Answer from the drawing. Dimensions are ordinates in mm from the lowest x, y and z of the part. A direction names the side the tool comes from. Give positions to 0.01 mm unless a question says otherwise; leave off trailing zeros. Order: outer loops, then holes, each group sorted by start corner. A loop starts at its lowest first (then second) coordinate and runs counter-clockwise, first axis right, second up. Notation, with made-up numbers: M 73.5,60.5 L 106.5,60.5 A10 ccw 106.5,75.5 Z; hole C -30,52.25 d7. An arc over 180 degrees is marked long. One line per item, written item: value.
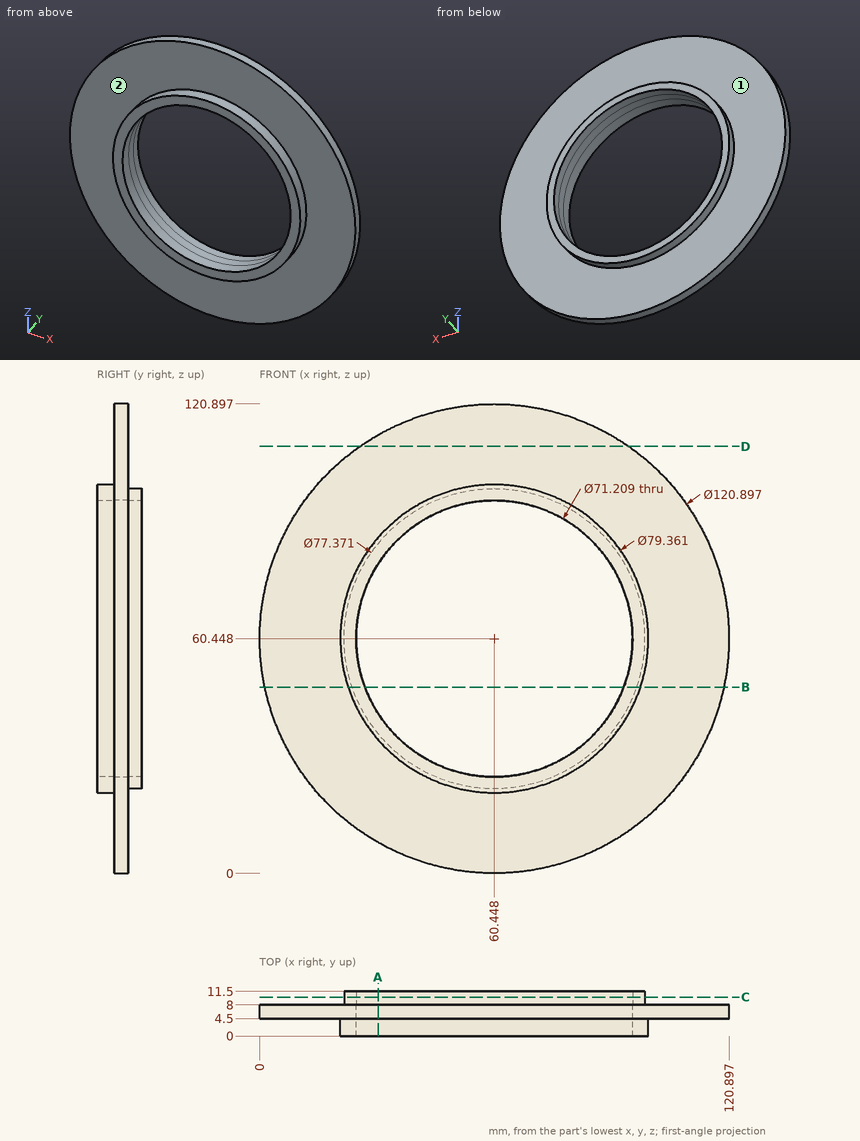
(1) Which of the six approach directions +Z, -Z, +X, -X, +Y, -Y give full straight-line access (tool end or side, diameter ignored) to the marked faces 1 and 2?
Findings:
face 1: +Y
face 2: -Y
(2) Section B-B, the plane z = 48 is taken. Give the vertices of the cut face in (x, y) (1 decimal), then the cut area to 3 significant figures.
Findings:
outline: M 1.3,4.5 L 22.8,4.5 L 22.8,0 L 27.1,0 L 27.1,11.5 L 23.8,11.5 L 23.8,8 L 1.3,8 Z; M 93.8,0 L 98.1,0 L 98.1,4.5 L 119.6,4.5 L 119.6,8 L 97.1,8 L 97.1,11.5 L 93.8,11.5 Z
area: 242 mm^2
(3) Section A-A, the plane x = 30.5 is taken. Give the vertices of the cut face in (y, z) (1 decimal).
Findings:
outline: M 0,34.4 L 4.5,34.4 L 4.5,7.9 L 8,7.9 L 8,36 L 11.5,36 L 11.5,41.2 L 0,41.2 Z; M 0,79.7 L 11.5,79.7 L 11.5,84.9 L 8,84.9 L 8,113 L 4.5,113 L 4.5,86.5 L 0,86.5 Z
(4) Section D-D, the plane z = 110 is taken. Give the vertices of the cut face in (x, y), then the cut area to 3 significant figures.
Findings:
outline: M 25.83,4.5 L 95.07,4.5 L 95.07,8 L 25.83,8 Z
area: 242 mm^2
(5) Section C-C, the plane y = 10 is taken. Give the vertices of the cut face in (x, z) (1 decimal), then the cut area to 3 significant figures.
Findings:
outline: C 60.4,60.4 d77.4; hole C 60.4,60.4 d71.2
area: 719 mm^2
(6) Find the intervals of material crossed by probe 1 along Z at (x, y) = (36, 1.25) (1 decimal); probe 2 along Z at (x, y) = (83.5, 6) (1 decimal); probe 3 along Y at (x, z) = (12, 40), in increasing order. Write a range as from..to.
Findings:
probe 1: z = 29.2..34.6, 86.3..91.7
probe 2: z = 4.6..33.3, 87.6..116.3
probe 3: y = 4.5..8
(7) Given P1, Ø3, axis at y = 9, z = 13, coming from the -X side; P2, Ø4, axis at x = 94, y = 3.5, coming from the +Z side (1 decimal); P3, Ø2, axis at x = 35.5, y = 8, coming from the +Z side, each flat-ended and moving along its own axis, determine where each tip first touches the part or whether it passes through.
Findings:
P1: stops at x = 21.62
P2: stops at z = 111.8
P3: stops at z = 115.95
